Check sheet for the modelled part. Datum: model origin and axes. Units: mm. A direction names the side the tool comes from. Round coordinates to 2 decimals unless told otherwise and drop trailing zeros. Order: outer loops, then holes, each group sorted by start corner. A loop starts at its lowest first (then second) coordinate and runs counter-clockwise, first axis right, second up. Notation, with made-up numbers: M 70.5,-3.5 L 76.5,-3.5 A8 ccw 76.5,6.5 Z; hole C 34,4.5 d10. An arc over 180 degrees is marked long. One line per item, written item: value. Start each with the question number.
(1) Release check for a two-part mould opening along Z. For faces 4 (the face through (17, 55, 10)), 5 (the face through (4, 30, 0)), 6 (the face through (15.524, 2.575, 6.632)) record: released by +Z, released by -Z, zero draft, split by the parting line, or undercut.
(2) Cross-section at A-A, the plane z = 10. Enter the section's corners in (x, y).
(3) Depth check by flat-ended pin: pin 1 Ø3 at (x, z) = (22, 14) entering from -Y; pin 2 Ø1.5 at (x, z) = (6, 9) entering from +Y; pin 3 Ø1 at (x, z) = (10, 15.5) entering from +Y; pin 4 Ø2.5 at (x, z) = (14, 14) entering from -Y. Enter the tip coordinate at first touch or a pass-through.
(4) Cross-section at D-D, the plane z = 17. Enter the section's corners in (x, y), and give its area (3 significant figures).
(5) Cross-section at C-C, the plane z = 14. Enter the section's corners in (x, y), and give its area (3 significant figures).
(6) Thickness scan on L1, parallel to Z at x = 22, y = 2.2; L2, parallel to X at y = 1.15, z = 14; L3, parallel to Y at x = 19.75, z = 3.5. Record the ranges inside material, lowest first.
(7) Access from +Z, -Z, +X, -X, +Y, -Y to the whole of each face (thin tool, end or side, straight path). Record for faces 1 (the face through (20, 57, 10)), 2 (the face through (15.574, 2.575, 13.504)), 3 (the face through (8.81, 53.09, 2.01)).
(8) Cross-section at B-B, the plane x = 22. Enter the section's corners in (y, z).
from build123d import *

# Parameters (mm, degrees)
BOSS_EXTRUDE1_DEPTH       = 20
FILLET1_R                 = 6.35
M4X0_7_TAPPED_HOLE1_D     = 3.3
M4X0_7_TAPPED_HOLE1_DEPTH = 10.1
M4X0_7_TAPPED_HOLE1_TIP   = 0.991420021
SKETCH5_R                 = 5.9563
CUT_EXTRUDE1_DEPTH        = 11.43


with BuildPart() as part:
    # Sketch1 → Boss-Extrude1 (new body)
    with BuildSketch(Plane.XY):
        Polygon((0, 0), (27, 0), (27, 5), (7, 5), (7, 55), (20, 55), (20, 60), (0, 60), align=None)
    extrude(amount=BOSS_EXTRUDE1_DEPTH)

    # Fillet1
    fillet1_edges = [part.edges().sort_by_distance(p)[0] for p in [
        (7, 55, 10),
        (7, 5, 10),
    ]]
    fillet(fillet1_edges, radius=FILLET1_R)

    # M4x0.7 Tapped Hole1
    with Locations(Plane(origin=(0, 0, 0), x_dir=(-1, 0, 0), z_dir=(0, -1, 0))):
        with Locations((-22, -14), (-22, -6), (-14, -6), (-14, -14)):
            Hole(M4X0_7_TAPPED_HOLE1_D / 2, depth=M4X0_7_TAPPED_HOLE1_DEPTH)
            with Locations((0, 0, -(M4X0_7_TAPPED_HOLE1_DEPTH + M4X0_7_TAPPED_HOLE1_TIP / 2))):  # 118° drill point
                Cone(0, M4X0_7_TAPPED_HOLE1_D / 2, M4X0_7_TAPPED_HOLE1_TIP, mode=Mode.SUBTRACT)

    # Sketch5 → Cut-Extrude1 (cut)
    with BuildSketch(Plane.XZ.offset(-60)):
        with Locations(Location((10, 10, 0), (0, 0, 120.242996609))):
            Circle(SKETCH5_R)
    extrude(amount=CUT_EXTRUDE1_DEPTH, mode=Mode.SUBTRACT)


solid = part.part
Values found:
1. face 4: zero draft
1. face 5: released by -Z
1. face 6: undercut
2. outline: M 0,0 L 27,0 L 27,5 L 13.35,5 A6.35 cw 7,11.35 L 7,48.57 L 4.04,48.57 L 4.04,60 L 0,60 Z; M 15.96,55 L 20,55 L 20,60 L 15.96,60 Z
3. pin 1: through
3. pin 2: y = 48.57
3. pin 3: y = 60
3. pin 4: y = 55
4. outline: M 0,0 L 27,0 L 27,5 L 13.35,5 A6.35 cw 7,11.35 L 7,48.65 A6.35 cw 13.35,55 L 20,55 L 20,60 L 0,60 Z
4. area: 602 mm^2
5. outline: M 0,0 L 12.35,0 L 12.35,5.08 A6.35 cw 7,11.35 L 7,48.57 L 5.59,48.57 L 5.59,60 L 0,60 Z; M 14.41,55 L 20,55 L 20,60 L 14.41,60 Z; M 15.65,0 L 20.35,0 L 20.35,5 L 15.65,5 Z; M 23.65,0 L 27,0 L 27,5 L 23.65,5 Z
5. area: 507 mm^2
6. L1: 0 to 4.35, 7.65 to 12.35, 15.65 to 20
6. L2: 0 to 12.35, 15.65 to 20.35, 23.65 to 27
6. L3: 0 to 5, 55 to 60
7. face 1: +Z, -Z, +X, +Y
7. face 2: -Y
7. face 3: +Z, -Z, +X
8. outline: M 0,0 L 5,0 L 5,4.35 L 0,4.35 Z; M 0,7.65 L 5,7.65 L 5,12.35 L 0,12.35 Z; M 0,15.65 L 5,15.65 L 5,20 L 0,20 Z
